```python
from build123d import *

# Parameters (mm, degrees)
SKETCH1_W           = 40.5
SKETCH1_H           = 20
BOSS_EXTRUDE1_DEPTH = 39
SKETCH2_R           = 3
BOSS_EXTRUDE2_DEPTH = 6
SKETCH3_W           = 2
SKETCH3_H           = 20
BOSS_EXTRUDE3_DEPTH = 7
SKETCH4_R           = 2
CUT_EXTRUDE1_DEPTH  = 7


with BuildPart() as part:
    # Sketch1 → Boss-Extrude1 (new body)
    with BuildSketch(Plane.XY):
        Rectangle(SKETCH1_W, SKETCH1_H)
    extrude(amount=BOSS_EXTRUDE1_DEPTH)

    # Sketch2 → Boss-Extrude2 (add)
    with BuildSketch(Plane.XY.offset(39)):
        with Locations((-10.25, 0)):
            Circle(SKETCH2_R)
    extrude(amount=BOSS_EXTRUDE2_DEPTH)

    # Sketch3 → Boss-Extrude3 (add)
    with BuildSketch(Plane.ZY.offset(20.25)):
        with Locations((30, 0)):
            Rectangle(SKETCH3_W, SKETCH3_H)
    boss_extrude3 = extrude(amount=BOSS_EXTRUDE3_DEPTH)

    # Sketch4 → Cut-Extrude1 (cut)
    with BuildSketch(Plane.XY.offset(31)):
        with Locations((-24.25, 6)):
            Circle(SKETCH4_R)
        with Locations(Location((-24.25, -6, 0), (0, 0, 270))):
            Circle(SKETCH4_R)
    cut_extrude1 = extrude(amount=-CUT_EXTRUDE1_DEPTH, mode=Mode.SUBTRACT)

    # Mirror1: Boss-Extrude3, Cut-Extrude1 across plane
    add(boss_extrude3.mirror(Plane(origin=(0, 0, 0), x_dir=(0, 0, 1), z_dir=(1, 0, 0))))
    add(cut_extrude1.mirror(Plane(origin=(0, 0, 0), x_dir=(0, 0, 1), z_dir=(1, 0, 0))), mode=Mode.SUBTRACT)


solid = part.part
```
Input: part model. Units: mm. Frame: model coordinates. A direction names the side the tool comes from. Round coordinates to 2 decimals unless told otherwise and drop trailing zeros. Loops run counter-clockwise (first coordinate to the right, second up) from the corner with the lowest first, then second, coordinate; pieces in that order, holes last. Notation, with made-up numbers: (79.5, -6) -> (101.5, -6) arc R23 cw to (101.5, 4) -> close; hole circle Ø5 at (-11, -2). An arc over 180 degrees is marked (long way). One line per item, written item: value.
(1) Section D-D (z = 22.5). Return the cut outline in (x, y), plus the area to 3 significant figures.
Geometry check:
outline: (-20.25, -10) -> (20.25, -10) -> (20.25, 10) -> (-20.25, 10) -> close
area: 810 mm2
(2) Section A-A (x = 24.25). Return the cut outline in (y, z), plus the area to 3 significant figures.
Geometry check:
outline: (-10, 29) -> (-8, 29) -> (-8, 31) -> (-10, 31) -> close; (-4, 29) -> (4, 29) -> (4, 31) -> (-4, 31) -> close; (8, 29) -> (10, 29) -> (10, 31) -> (8, 31) -> close
area: 24.0 mm2
(3) Pin query (flat end, axial travel): pin 1 (3 mm diameter, centred on y = 0.5, z = 22.5, fed in from -X); pin 2 (2.5 mm diameter, centred on y = 3.5, z = 35, fed in from +X); pin 3 (8 mm diameter, centred on x = 6.5, y = -4.5, fed in from +Z). Return the tip coordinate at first contact, or that it passes through.
Geometry check:
pin 1: x = -20.25
pin 2: x = 20.25
pin 3: z = 39
(4) Section C-C (x = -10.25). Return the cut outline in (y, z), plus the area to 3 significant figures.
Geometry check:
outline: (-10, 0) -> (10, 0) -> (10, 39) -> (3, 39) -> (3, 45) -> (-3, 45) -> (-3, 39) -> (-10, 39) -> close
area: 816 mm2
(5) Set-up query: faces 4 (the face through (20.25, 0, 14)), 5 (the face through (-24, 0, 29)), 6 (the face through (-24, 0, 31)), 7 (the face through (-12.631, -1.825, 41.958)). Return all of +Z, -Z, +X, -X, +Y, -Y with unobstructed straight access to the full face (end or side cutting, diameter ignored); none if empty.
Geometry check:
face 4: -Z, +X, +Y, -Y
face 5: -Z, -X, +Y, -Y
face 6: +Z, -X, +Y, -Y
face 7: +Z
(6) Material intervals for line 1 (Y direction, x = 24.25, z = 30.05); line 2 (X direction, y = -6, z = 30.4); line 3 (X direction, y = -6, z = 22), sorted ascending. Write a range as [from, to].
Geometry check:
line 1: [-10, -8], [-4, 4], [8, 10]
line 2: [-27.25, -26.25], [-22.25, 22.25], [26.25, 27.25]
line 3: [-20.25, 20.25]
(7) Mould query, pull axis Y, two halves, no side actions, for faces 1 (the face through (0, -10, 19)), 2 (the face through (26.248, 6.088, 30.014)), 3 (the face through (24, 0, 29)). Classes: pulls with the +Y half, pulls with the -Y half, needs draft (parallel to the pull), parting line crosses it, or undercut.
Geometry check:
face 1: pulls with the -Y half
face 2: undercut
face 3: needs draft
(8) Section B-B (y = -6). Return the cut outline in (x, z), plus the area to 3 significant figures.
Geometry check:
outline: (-27.25, 29) -> (-26.25, 29) -> (-26.25, 31) -> (-27.25, 31) -> close; (-22.25, 29) -> (-20.25, 29) -> (-20.25, 0) -> (20.25, 0) -> (20.25, 29) -> (22.25, 29) -> (22.25, 31) -> (20.25, 31) -> (20.25, 39) -> (-20.25, 39) -> (-20.25, 31) -> (-22.25, 31) -> close; (26.25, 29) -> (27.25, 29) -> (27.25, 31) -> (26.25, 31) -> close
area: 1,590 mm2
